```python
from build123d import *

# Parameters (mm, degrees)
SKETCH_1_R                        = 6.5
EXTRUDE_1_DEPTH                   = 40
SKETCH_2_W                        = 15
SKETCH_2_H                        = 60
SKETCH_3_W                        = 12
SKETCH_3_H                        = 60
EXTRUDE_2_DEPTH                   = 15
CUT_EXTRUDE_1_DEPTH               = 21.0000001
HOLE_WIZARD_2_8_2_8_1_D           = 2.8
HOLE_WIZARD_2_8_2_8_1_CSINK_D     = 2.85
HOLE_WIZARD_2_8_2_8_1_CSINK_ANGLE = 90


with BuildPart() as part:
    # 草圖1 → 填料-伸長1 (new body)
    with BuildSketch(Plane.XY):
        with BuildLine():
            Line((15, 14), (0, 14))
            ThreePointArc((0, 14), (-14, 0), (0, -14))
            Line((0, -14), (15, -14))
            Line((15, -14), (15, 14))
        make_face()
        Circle(SKETCH_1_R, mode=Mode.SUBTRACT)
    extrude(amount=EXTRUDE_1_DEPTH)

    # 草圖2 → section 1 of loft_1
    with BuildSketch(Plane(origin=(84.27, 0, 0), x_dir=(0, 0, -1), z_dir=(1, 0, 0)), mode=Mode.PRIVATE) as loft_1_s1:
        with Locations((-12.5, 0)):
            Rectangle(SKETCH_2_W, SKETCH_2_H)
    # loft from a face of the part (loft_1)
    loft([part.faces().sort_by_distance((15, 0, 20))[0], loft_1_s1.sketch])

    # 草圖3 → 填料-伸長2 (add)
    with BuildSketch(Plane(origin=(84.27, 0, 0), x_dir=(0, 0, -1), z_dir=(1, 0, 0))):
        with Locations((-14, 0)):
            Rectangle(SKETCH_3_W, SKETCH_3_H)
    extrude(amount=EXTRUDE_2_DEPTH)

    # 草圖4 → 除料-伸長1 (cut, through all)
    with BuildSketch(Plane.XY.offset(20)):
        with BuildLine():
            Line((91.27, 25), (91.27, 15))
            ThreePointArc((91.27, 15), (89.27, 13), (87.27, 15))
            Line((87.27, 15), (87.27, 25))
            ThreePointArc((87.27, 25), (89.27, 27), (91.27, 25))
        make_face()
        with BuildLine():
            Line((91.27, -15), (91.27, -25))
            ThreePointArc((91.27, -25), (89.27, -27), (87.27, -25))
            Line((87.27, -25), (87.27, -15))
            ThreePointArc((87.27, -15), (89.27, -13), (91.27, -15))
        make_face()
    extrude(amount=-CUT_EXTRUDE_1_DEPTH, mode=Mode.SUBTRACT)

    # Ø2.8 (2.8) 直徑孔1 (through all)
    with Locations(Plane(origin=(0, 14, 0), x_dir=(1, 0, 0), z_dir=(0, 1, 0))):
        with Locations((0, -20)):
            CounterSinkHole(HOLE_WIZARD_2_8_2_8_1_D / 2, HOLE_WIZARD_2_8_2_8_1_CSINK_D / 2, counter_sink_angle=HOLE_WIZARD_2_8_2_8_1_CSINK_ANGLE)


solid = part.part
```
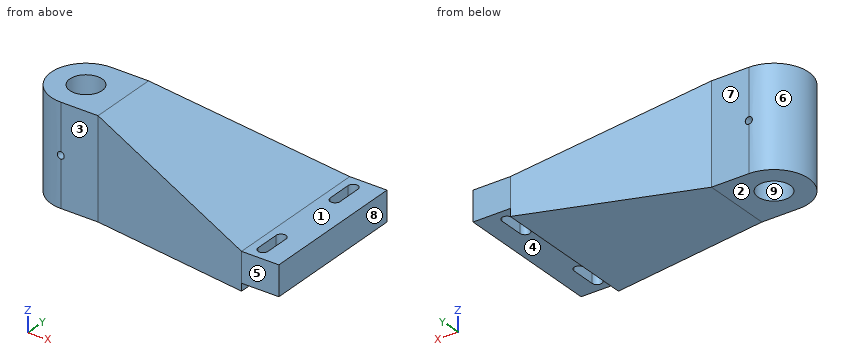
The listing builds one solid part. Answer for the finished solid, in the listing's coordinates (mm). Face numbers are marked on the shaded views. A direction names the side the tool comes from. Give positions to 0.01 mm unless a question says otherwise; leave off trailing zeros. Loops run counter-clockwise (first coordinate to the right, second up) from the corner with the lowest first, then second, coordinate; pieces in that order, holes last. Notation, with made-up numbers: (74, 14.5) - (97, 14.5) arc R25 ccw to (97, 33.5) - close; hole circle Ø6 at (18, 86). An arc over 180 degrees is marked (long way). Answer as CSV lines item,"result". Start each with the question number.
Item 1: A cutting plane is placed at A-A on x = 89.27. Determine the outline of the cut face in (y, z).
Item 2: For the marked faces 1, 2, 3, 4 and 5, determine the directions among +Z, -Z, +X, -X, +Y, -Y from which every point of the face is accessible in a straight line to the end or side of a thin tool.
Item 3: Each of these flat-tipped pins is pushed along its axis until it touches: pin 1 (1 mm diameter, centred on x = 32.5, z = 17.5, fed in from -Y); pin 2 (2 mm diameter, centred on x = 30, z = 32.5, fed in from -Y); pin 3 (4.5 mm diameter, centred on x = 8, z = 20.5, fed in from +Y); pin 4 (1.7 mm diameter, centred on x = 0, z = 20, fed in from +Y). Where does it stop, or does it pass through?
Item 4: Find the intervals of material crossed by line 1 (Z direction, x = 0, y = -9.5); line 2 (Z direction, x = 93, y = 10.5); line 3 (Y direction, x = 88, z = 12.5), in increasing order. Write a range as from..to.
Item 5: A cutting plane is placed at B-B on x = 3. Determine the outline of the cut face in (y, z).
Item 6: The mould has two halves that part along X. Classify the marked faces 6, 7, 8 and 9: +X half, -X half, draft (parallel to the pull), parting line (faces both ways), or undercut.
Found:
1,outline,"(-30, 8) - (-27, 8) - (-27, 20) - (-30, 20) - close; (-13, 8) - (13, 8) - (13, 20) - (-13, 20) - close; (27, 8) - (30, 8) - (30, 20) - (27, 20) - close"
2,face 1,"+Z, +X, +Y, -Y"
2,face 2,"-Z, +X, -X, +Y, -Y"
2,face 3,"+Z, -Z, -X, -Y"
2,face 4,"-Z, +X, +Y, -Y"
2,face 5,"+Z, -Z, +X, -X, -Y"
3,pin 1,"stops at y = -18.16"
3,pin 2,"stops at y = -17.7"
3,pin 3,"stops at y = 14"
3,pin 4,"passes through"
4,line 1,"z = 0..18.6, 21.4..40"
4,line 2,"z = 8..20"
4,line 3,"y = -30..-26.55, -13.45..13.45, 26.55..30"
5,outline,"(-14, 0) - (-5.77, 0) - (-5.77, 40) - (-14, 40) - close; (5.77, 0) - (14, 0) - (14, 40) - (5.77, 40) - close"
6,face 6,"-X half"
6,face 7,"draft"
6,face 8,"+X half"
6,face 9,"undercut"
